```python
from build123d import *

# Parameters (mm, degrees)
SKETCH1_W               = 47.625
SKETCH1_H               = 47.625
BOSS_EXTRUDE1_DEPTH     = 15.875
SKETCH2_R               = 19.05
BOSS_EXTRUDE2_DEPTH     = 3.175
SKETCH3_R               = 14.2875
CUT_EXTRUDE1_DEPTH      = 20.05
F_1_4_20_TAPPED_HOLE1_D = 5.1054
FILLET1_R               = 6.35


with BuildPart() as part:
    # Sketch1 → Boss-Extrude1 (new body)
    with BuildSketch(Plane(origin=(0, 0, 0), x_dir=(1, 0, 0), z_dir=(0, 1, 0))):
        Rectangle(SKETCH1_W, SKETCH1_H)
    extrude(amount=BOSS_EXTRUDE1_DEPTH)

    # Sketch2 → Boss-Extrude2 (add)
    with BuildSketch(Plane(origin=(0, 15.875, 0), x_dir=(1, 0, 0), z_dir=(0, 1, 0))):
        Circle(SKETCH2_R)
    extrude(amount=BOSS_EXTRUDE2_DEPTH)

    # Sketch3 → Cut-Extrude1 (cut, through all)
    with BuildSketch(Plane(origin=(0, 19.05, 0), x_dir=(1, 0, 0), z_dir=(0, 1, 0))):
        Circle(SKETCH3_R)
    extrude(amount=-CUT_EXTRUDE1_DEPTH, mode=Mode.SUBTRACT)

    # 1/4-20 Tapped Hole1 (through all)
    with Locations(Plane(origin=(0, 15.875, 0), x_dir=(1, 0, 0), z_dir=(0, 1, 0))):
        with Locations((-17.4625, 17.4625), (17.4625, 17.4625), (17.4625, -17.4625), (-17.4625, -17.4625)):
            Hole(F_1_4_20_TAPPED_HOLE1_D / 2)

    # Fillet1
    fillet1_edges = [part.edges().sort_by_distance(p)[0] for p in [
        (-23.8125, 7.9375, -23.8125),
        (23.8125, 7.9375, -23.8125),
        (23.8125, 7.9375, 23.8125),
        (-23.8125, 7.9375, 23.8125),
    ]]
    fillet(fillet1_edges, radius=FILLET1_R)


solid = part.part
```
The listing builds one solid part. Answer for the finished solid, in the listing's coordinates (mm). A direction names the side the tool comes from. Round coordinates to 2 decimals unless told otherwise and drop trailing zeros. Use CSV: the item, a comma, the result in double quotes. Start each with the question number.
(1) Which of the six approach directions +Z, -Z, +X, -X, +Y, -Y give full straight-line access (tool end or side, diameter ignored) to faces 1 (the face through (-22.002, 8.049, 21.903)), 2 (the face through (-15.12, 17.44, 11.59))?
(2) The mould has two halves that part along Z. Classify faces 3 (the face through (-14.274, 9.658, -0.628)), 4 (the face through (21.903, 8.049, 22.002)), 5 (the face through (-22.002, 8.049, -21.903)): released by +Z, released by -Z, zero draft, split by the parting line, or undercut.
(3) Section C-C on y = 9 is taken. Count the separate pieces of the cut face and the enclosed holes in it, then the cut area to 3 significant figures.
(4) Consider L1, parallel to Z at x = 17.5, y = 8.75; L2, parallel to Z at x = 15.5, y = 6.75; L3, parallel to Y at x = -11, z = 21.5 (3 decimals). Determine where each line is inside the solid, lowest interval first. Write a range as from..to.
(5) This flat-tipped pin is pushed along its axis until it touches: pin 1 (8 mm diameter, centred on x = 17.46, z = 17.46, fed in from +Y) (3 decimals). Where does it stop, or does it pass through?
A:
1,face 1,"+Z, -X, +Y, -Y"
1,face 2,"+Y"
2,face 3,"undercut"
2,face 4,"released by +Z"
2,face 5,"released by -Z"
3,separate pieces,"1"
3,enclosed holes,"5"
3,area,"1,510 mm²"
4,L1,"z = -23.81..-20.01, -14.91..14.91, 20.01..23.81"
4,L2,"z = -23.81..-19.09, -15.83..15.83, 19.09..23.81"
4,L3,"y = 0..15.875"
5,pin 1,"stops at y = 15.875"
